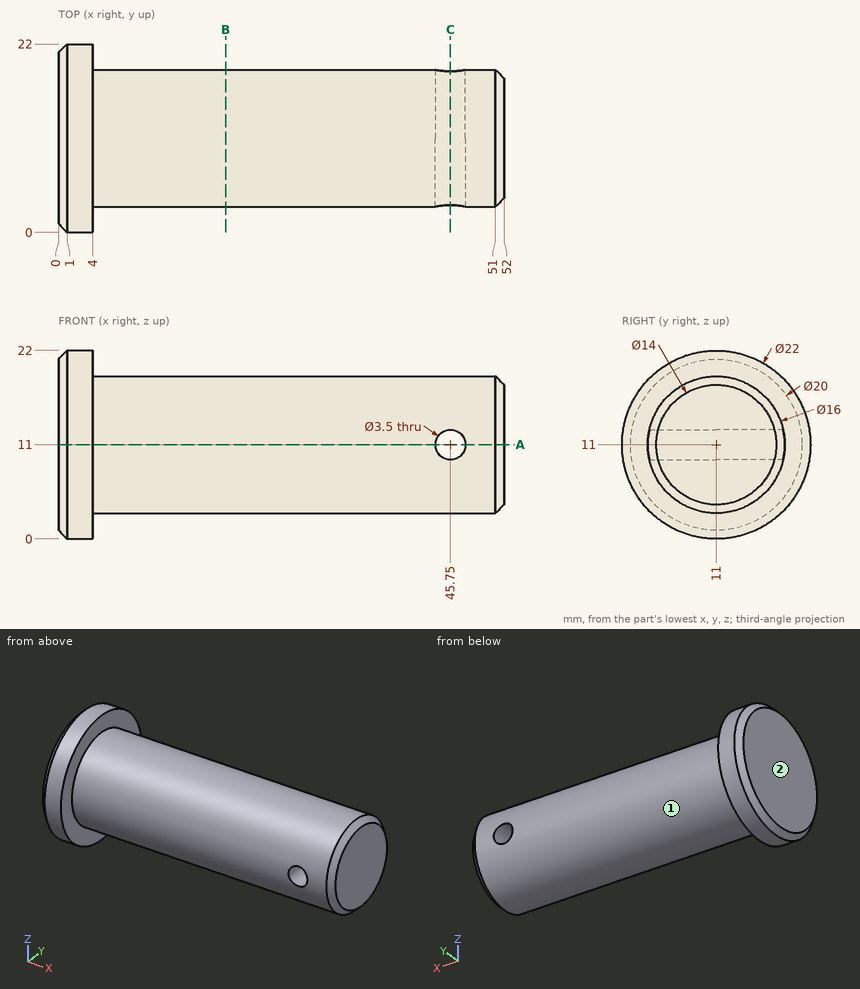
Here's the drawing with two shaded views (mm, measured from the low corner). I have some questions. A direction names the side the tool comes from. Coordinates: 2 decimals unless noted, no trailing zeros. Loops run counter-clockwise (first coordinate to the right, second up) from the corner with the lowest first, then second, coordinate; pieces in that order, holes last. Notation, with made-up numbers: (-20, 56.25) -> (-7, 56.25) arc R3 ccw to (-7, 60.25) -> close; hole circle Ø11 at (3, 74). An arc over 180 degrees is marked (long way). Put each result on its own line as item: value. Start each with the question number.
Q1. For the marked faces 1 and 2, which set-ups out of +Z, -Z, +X, -X, +Y, -Y let a thin tool reach every point of the face, with its end or its side?
Q2. If I drill on line 1 (X direction, y = 13.5, z = 11); line 2 (X direction, y = 16.75, z = 19); line 3 (Z direction, x = 45.75, y = 4.75), over which ranges is the centre line in solid material (lowest first)? Write a range as [from, to].
Q3. I want a section at C-C (x = 45.75). Write out the boundary of the cut face in (y, z), plus the area to 3 significant figures.
Q4. I want a section at B-B (x = 19.5). Write out the boundary of the cut face in (y, z).
Q5. I want a section at A-A (z = 11). Write out the boundary of the cut face in (x, y), plus the area to 3 significant figures.
Q6. I'm going to push flat-ended pins straight in: P1, Ø3, axis at x = 21.5, y = 14.5, coming from the -Z side; P2, Ø6, axis at x = 24, y = 19, coming from the +Z side (3 decimals); P3, Ø3, axis at x = 37, y = 10.5, coming from the +Z side. Where does each tip first touch, or does it pass through?
Taken from the geometry:
1. face 1: +X
1. face 2: +Z, -Z, -X, +Y, -Y
2. line 1: x = [0, 44], [47.5, 52]
2. line 2: x = [0, 4]
2. line 3: z = [6.01, 9.25], [12.75, 15.99]
3. outline: (3.19, 9.25) arc R8 ccw to (18.81, 9.25) -> close; (3.19, 12.75) -> (18.81, 12.75) arc R8 ccw to start
3. area: 146 mm2
4. outline: circle Ø16 at (11, 11)
5. outline: (0, 1) -> (1, 0) -> (4, 0) -> (4, 3) -> (44, 3) -> (44, 19) -> (4, 19) -> (4, 22) -> (1, 22) -> (0, 21) -> close; (47.5, 3) -> (51, 3) -> (52, 4) -> (52, 18) -> (51, 19) -> (47.5, 19) -> close
5. area: 798 mm2
6. P1: stops at z = 3.25
6. P2: stops at z = 17.245
6. P3: stops at z = 19
